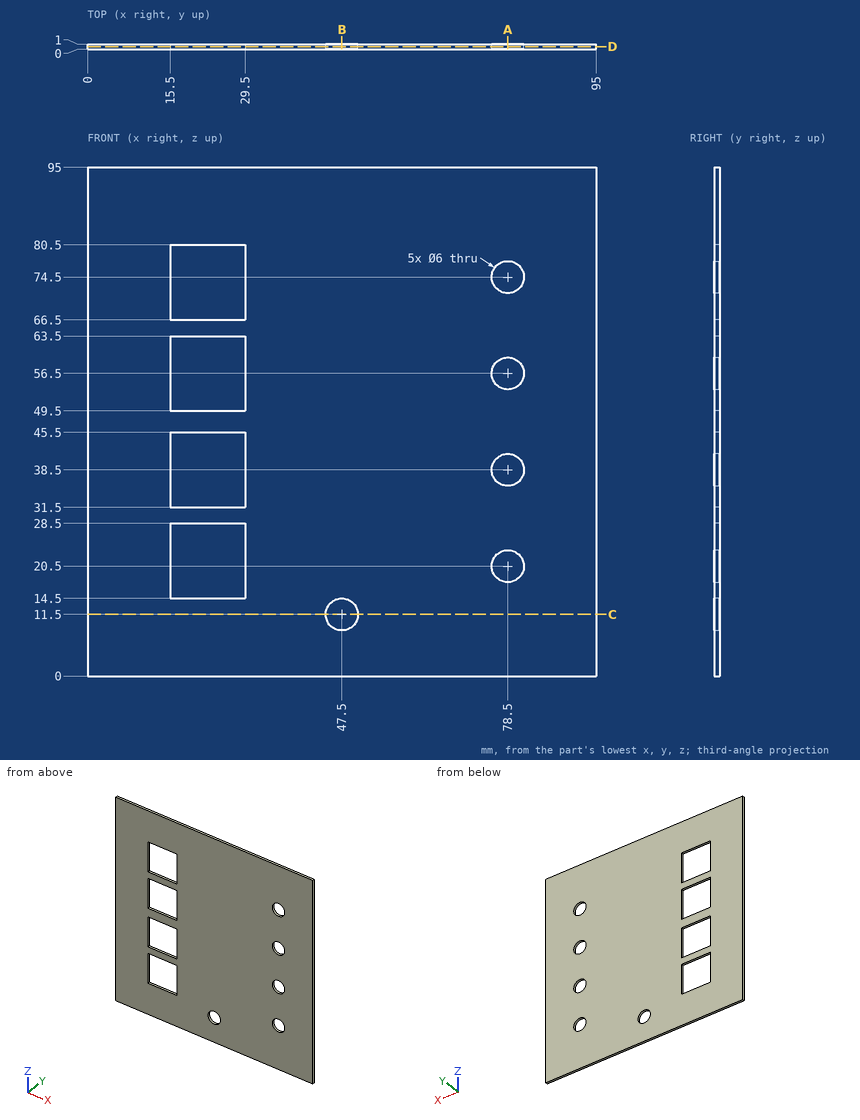
Drawing for the job (mm, zero at the part's lowest x, y, z). Round coordinates to 2 decimals unless told otherwise and drop trailing zeros. Write each loop counter-clockwise with the first axis right and the second up, starting at its lowest first coordinate (ties: lowest second). Pieces come first, ordered by that corner, then holes. Notation, with made-up numbers: M 44,61.5 L 89,61.5 A15 ccw 89,78.5 Z; hole C -15,1 d2. An arc over 180 degrees is marked long. One line per question, with ' | ' between items.
1. Probe L1, parallel to X at y = 0.65, z = 38.5; L2, parallel to Z at x = 21.5, y = 0.6; L3, parallel to X at y = 0.5, z = 43.5. List the from-to ranges inside material, lowest first. Write a range as from..to.
Working result:
L1: 0..15.5, 29.5..75.5, 81.5..95 | L2: 0..14.5, 28.5..31.5, 45.5..49.5, 63.5..66.5, 80.5..95 | L3: 0..15.5, 29.5..95
2. Cut at B-B on x = 47.5. Write the cut outline in (y, z).
Working result:
outline: M 0,0 L 1,0 L 1,8.5 L 0,8.5 Z; M 0,14.5 L 1,14.5 L 1,95 L 0,95 Z
3. Pin check, flat tip, straight feed: pin 1 Ø6 at (x, z) = (27.5, 73) entering from -Y. Stop position of the tip, or through.
Working result:
pin 1: y = 0
4. Cut at C-C on z = 11.5. Write the cut outline in (x, y).
Working result:
outline: M 0,0 L 44.5,0 L 44.5,1 L 0,1 Z; M 50.5,0 L 95,0 L 95,1 L 50.5,1 Z
5. Cut at D-D on y = 0.5. Count the separate pieces of the cut face and the enclosed holes in it, and give its area (3 significant figures).
Working result:
separate pieces: 1 | enclosed holes: 9 | area: 8,100 mm2
6. Cut at A-A on x = 78.5. Write the cut outline in (y, z).
Working result:
outline: M 0,0 L 1,0 L 1,17.5 L 0,17.5 Z; M 0,23.5 L 1,23.5 L 1,35.5 L 0,35.5 Z; M 0,41.5 L 1,41.5 L 1,53.5 L 0,53.5 Z; M 0,59.5 L 1,59.5 L 1,71.5 L 0,71.5 Z; M 0,77.5 L 1,77.5 L 1,95 L 0,95 Z
